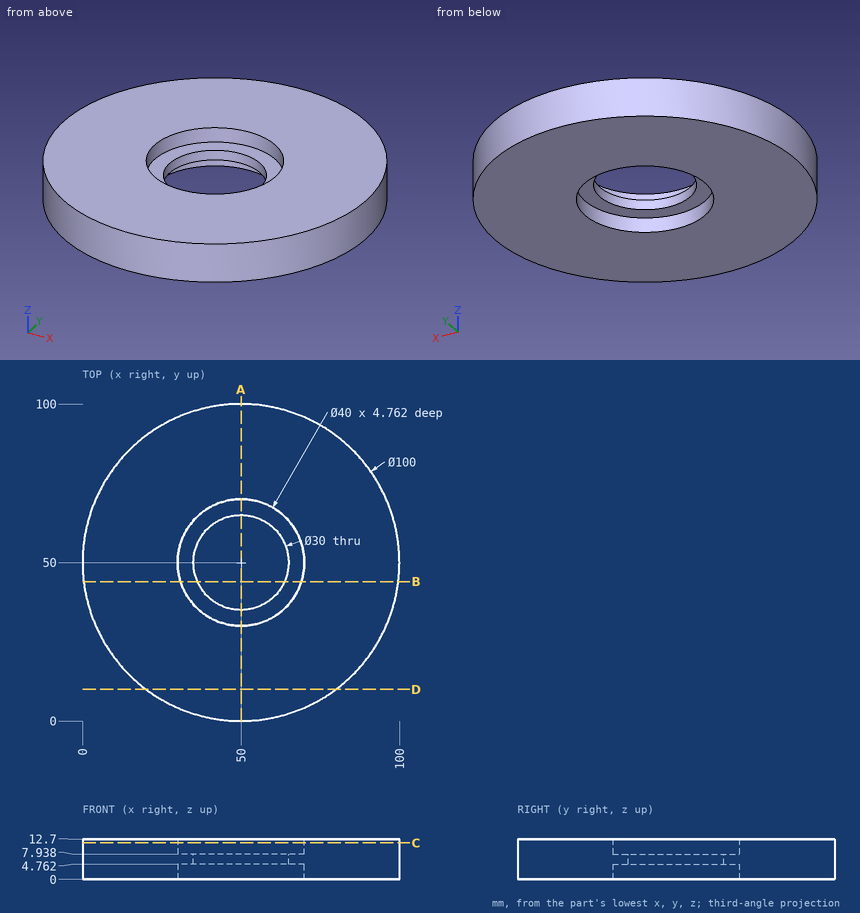
Design review of the part shown in the three views and the two pictorial views. Dimensions are in mm from the part's minimum x, y and z. Round coordinates to 2 decimals unless told otherwise and drop trailing zeros. Loops run counter-clockwise (first coordinate to the right, second up) from the corner with the lowest first, then second, coordinate; pieces in that order, holes last.
1) Clearance check with flat-ended pins moving along their axes: P1, Ø2, axis at x = 27.5, z = 8.5, coming from the -Y side; P2, Ø4, axis at x = 89.5, z = 10.5, coming from the -Y side; P3, Ø2, axis at x = 82.5, z = 3, coming from the +Y side. State where each tip first meets the part, or that it passes through.
Values follow:
P1: stops at y = 4.86
P2: stops at y = 16.93
P3: stops at y = 88.83
2) Consider section C-C on z = 11.5. State the section outline as (x, y) points, then the cut area to 3 significant figures.
Values follow:
outline: circle Ø100 at (50, 50); hole circle Ø40 at (50, 50)
area: 6,600 mm2
3) Consider section A-A on x = 50. State the section outline as (y, z) points.
Values follow:
outline: (0, 0) - (30, 0) - (30, 4.76) - (35, 4.76) - (35, 7.94) - (30, 7.94) - (30, 12.7) - (0, 12.7) - close; (65, 4.76) - (70, 4.76) - (70, 0) - (100, 0) - (100, 12.7) - (70, 12.7) - (70, 7.94) - (65, 7.94) - close
4) Wall thickness on line 1 along Y through (x, z) = (50, 11.3); line 2 along Y through (x, z) = (50, 5.5); line 3 along X through (y, z) = (44, 9.25): over which ranges is each line inside the solid? List them lowest first.
Values follow:
line 1: y = 0 to 30, 70 to 100
line 2: y = 0 to 35, 65 to 100
line 3: x = 0.36 to 30.92, 69.08 to 99.64
5) Consider section D-D on y = 10. State the section outline as (x, z) points, then the cut area to 3 significant figures.
Values follow:
outline: (20, 0) - (80, 0) - (80, 12.7) - (20, 12.7) - close
area: 762 mm2
6) Consider section B-B on y = 44. State the section outline as (x, z) points, then the cut area to 3 significant figures.
Values follow:
outline: (0.36, 0) - (30.92, 0) - (30.92, 4.76) - (36.25, 4.76) - (36.25, 7.94) - (30.92, 7.94) - (30.92, 12.7) - (0.36, 12.7) - close; (63.75, 4.76) - (69.08, 4.76) - (69.08, 0) - (99.64, 0) - (99.64, 12.7) - (69.08, 12.7) - (69.08, 7.94) - (63.75, 7.94) - close
area: 810 mm2
